Build history of the part. All positions in model axes, mm. Face numbers are marked on the shaded views. A direction names the side the tool comes from. Round coordinates to 2 decimals unless told otherwise and drop trailing zeros. Write each loop counter-clockwise with the first axis right and the second up, starting at its lowest first coordinate (ties: lowest second). Pieces come first, ordered by that corner, then holes. Notation, with made-up numbers: M 46,-2 L 73,-2 A16 cw 73,22 Z; hole C 36,59.5 d6. An arc over 180 degrees is marked long. Use a Markdown table: item, result.
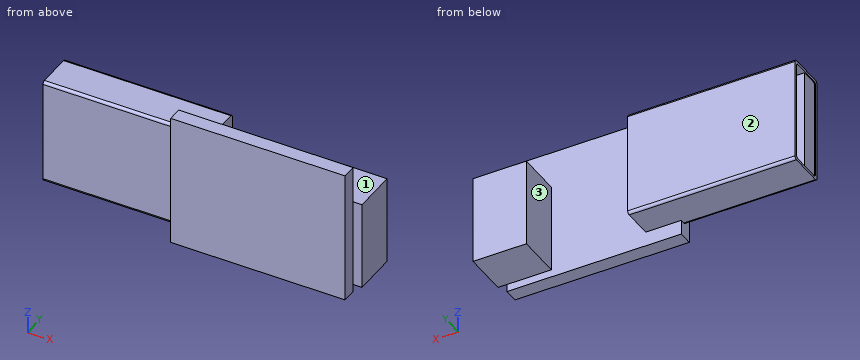
from build123d import *

# Parameters (mm, degrees)
SKETCH1_W           = 19.6
SKETCH1_H           = 15
BOSS_EXTRUDE1_DEPTH = 0.8
SKETCH2_W           = 18.8
SKETCH2_H           = 12
BOSS_EXTRUDE2_DEPTH = 4.4
SKETCH3_W           = 11.4
SKETCH3_H           = 3.8
CUT_EXTRUDE1_DEPTH  = 16.8
FILLET1_R           = 0.3
SKETCH4_W           = 6
SKETCH4_H           = 10
BOSS_EXTRUDE3_DEPTH = 5
BOSS_EXTRUDE4_DEPTH = 16.7


with BuildPart() as part:
    # Sketch1 → Boss-Extrude1 (new, symmetric)
    with BuildSketch(Plane(origin=(0, 0, 0), x_dir=(1, 0, 0), z_dir=(0, 1, 0))):
        Rectangle(SKETCH1_W, SKETCH1_H)
    extrude(amount=BOSS_EXTRUDE1_DEPTH, both=True)

    # Sketch2 → Boss-Extrude2 (add)
    with BuildSketch(Plane(origin=(0, 0, 0), x_dir=(1, 0, 0), z_dir=(0, 1, 0))):
        with Locations((-15.2, -0.15)):
            Rectangle(SKETCH2_W, SKETCH2_H)
    extrude(amount=BOSS_EXTRUDE2_DEPTH)

    # Sketch3 → Cut-Extrude1 (cut)
    with BuildSketch(Plane.ZY.offset(24.6)):
        with Locations((0.15, 2.2)):
            Rectangle(SKETCH3_W, SKETCH3_H)
    extrude(amount=-CUT_EXTRUDE1_DEPTH, mode=Mode.SUBTRACT)

    # Fillet1
    fillet1_edges = [part.edges().sort_by_distance(p)[0] for p in [
        (-17.2, 0, 6.15),
        (-17.2, 0, -5.85),
        (-15.2, 4.4, 6.15),
        (-15.2, 4.4, -5.85),
        (-16.2, 0.3, 5.85),
        (-16.2, 0.3, -5.55),
        (-16.2, 4.1, -5.55),
        (-16.2, 4.1, 5.85),
    ]]
    fillet(fillet1_edges, radius=FILLET1_R)

    # Sketch4 → Boss-Extrude3 (add)
    with BuildSketch(Plane(origin=(0, 0.8, 0), x_dir=(1, 0, 0), z_dir=(0, 1, 0))):
        with Locations((7.8, 1.65)):
            Rectangle(SKETCH4_W, SKETCH4_H)
    extrude(amount=BOSS_EXTRUDE3_DEPTH)

    # Sketch5 → Boss-Extrude4 (add)
    with BuildSketch(Plane.ZY.offset(7.8)):
        with BuildLine():
            Line((5.55, 0.3), (-5.25, 0.3))
            ThreePointArc((-5.25, 0.3), (-5.462132034, 0.387867966), (-5.55, 0.6))
            Line((-5.55, 0.6), (-5.55, 2.3))
            Line((-5.55, 2.3), (5.85, 2.3))
            Line((5.85, 2.3), (5.85, 0.6))
            ThreePointArc((5.85, 0.6), (5.762132034, 0.387867966), (5.55, 0.3))
        make_face()
    extrude(amount=BOSS_EXTRUDE4_DEPTH)


solid = part.part
Q1. Cut at C-C on z = -0.5. Give the cut face in (x, y).
Response values:
| item | result |
|---|---|
| outline | M -24.6,0 L -9.8,0 L -9.8,-0.8 L 9.8,-0.8 L 9.8,0.8 L 10.8,0.8 L 10.8,5.8 L 4.8,5.8 L 4.8,0.8 L -5.8,0.8 L -5.8,4.4 L -24.6,4.4 L -24.6,4.1 L -7.8,4.1 L -7.8,2.3 L -24.5,2.3 L -24.5,0.3 L -24.6,0.3 Z |
Q2. Cut at A-A on x = -21.5. Give the cut face in (y, z).
Response values:
| item | result |
|---|---|
| outline | M 0,-5.55 A0.3 ccw 0.3,-5.85 L 4.1,-5.85 A0.3 ccw 4.4,-5.55 L 4.4,5.85 A0.3 ccw 4.1,6.15 L 0.3,6.15 A0.3 ccw 0,5.85 Z; hole M 2.3,-5.55 L 3.8,-5.55 A0.3 ccw 4.1,-5.25 L 4.1,5.55 A0.3 ccw 3.8,5.85 L 2.3,5.85 Z |
Q3. Drop flat-ended pins along their axis: P1, Ø1.5, axis at x = 7.5, y = 3, coming from the +Z side; P2, Ø3.5, axis at x = -19, y = 1.5, coming from the -Z side; P3, Ø3, axis at x = -17.5, z = -3, coming from the +Y side; P4, Ø2, axis at x = -4.5, y = 3.5, coming from the +Z side. Give the stop position or say it passes through.
Response values:
| item | result |
|---|---|
| P1 | stops at z = 3.35 |
| P2 | stops at z = -5.85 |
| P3 | stops at y = 4.4 |
| P4 | passes through |
Q4. Cut at B-B on y = 3. Give the cut face in (x, z), and give its area (3 significant figures).
Response values:
| item | result |
|---|---|
| outline | M -24.6,-5.85 L -5.8,-5.85 L -5.8,6.15 L -24.6,6.15 L -24.6,5.85 L -7.8,5.85 L -7.8,-5.55 L -24.6,-5.55 Z; M 4.8,-6.65 L 10.8,-6.65 L 10.8,3.35 L 4.8,3.35 Z |
| area | 94.1 mm2 |
Q5. Drill centre lines: L1, parallel to X at y = 1.25, z = -1.5; L2, parallel to Z at x = -12, y = 3; L3, parallel to Y at x = -13, z = -3.5. Where is each one in solid material? Low to high.
Response values:
| item | result |
|---|---|
| L1 | x = -24.5 to -5.8, 4.8 to 10.8 |
| L2 | z = -5.85 to -5.55, 5.85 to 6.15 |
| L3 | y = 0 to 2.3, 4.1 to 4.4 |
Q6. Cut at D-D on z = 4.75. Give the cut face in (x, y), and give its area (3 significant figures).
Response values:
| item | result |
|---|---|
| outline | M -24.6,0 L -9.8,0 L -9.8,-0.8 L 9.8,-0.8 L 9.8,0.8 L -5.8,0.8 L -5.8,4.4 L -24.6,4.4 L -24.6,4.1 L -7.8,4.1 L -7.8,2.3 L -24.5,2.3 L -24.5,0.3 L -24.6,0.3 Z |
| area | 80.4 mm2 |
Q7. Which spindle directions (+Z, -Z, +X, -X, +Y, -Y) get a long thin tool onto all of the face, cutting with end or side? Do the marked faces 1, 2 and 3. Say none if no direction does.
Response values:
| item | result |
|---|---|
| face 1 | +Z, +X, +Y |
| face 2 | +Z, -Z, -X, +Y |
| face 3 | +Z, -Z, +Y |
